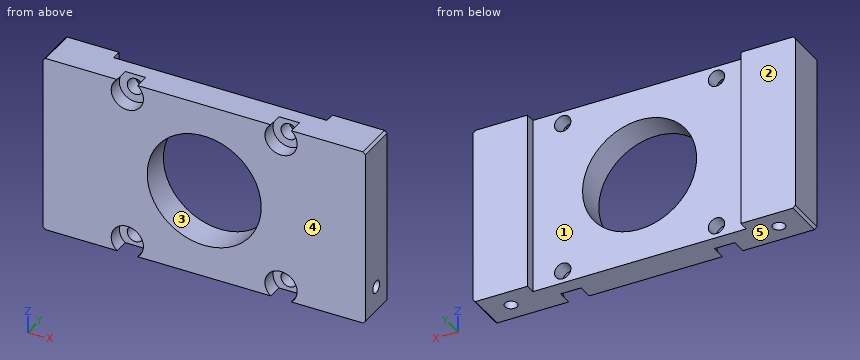
from build123d import *

# Parameters (mm, degrees)
F0_W           = 65
F0_H           = 36
F0_R           = 11.5
F1_DEPTH       = 8
F3_D           = 3.3
F3_CBORE_D     = 6.5
F3_CBORE_DEPTH = 3
F4_SIZE        = 0.5
F6_D           = 2.5
F6_DEPTH       = 13.5
F6_TIP         = 0.7510757738
F7_W           = 43
F7_H           = 36
F7_R           = 1.65
F7_R_2         = 11.5
F8_DEPTH       = 2
F10_D          = 2.5
F10_DEPTH      = 13.5
F10_TIP        = 0.7510757738


with BuildPart() as f1:
    # F0 (on Front) → F1 (new body)
    with BuildSketch(Plane.XZ):
        Rectangle(F0_W, F0_H)
        Circle(F0_R, mode=Mode.SUBTRACT)
    extrude(amount=F1_DEPTH)

    # F3 (through all)
    with Locations(Plane.XZ.offset(8)):
        with Locations((15.5, 15.5), (15.5, -15.5), (-15.5, -15.5), (-15.5, 15.5)):
            CounterBoreHole(F3_D / 2, F3_CBORE_D / 2, F3_CBORE_DEPTH)

    # F4
    f4_edges = [f1.edges().sort_by_distance(p)[0] for p in [
        (-32.5, -4, 18),
        (32.5, -4, 18),
        (32.5, -4, -18),
        (-32.5, -4, -18),
    ]]
    chamfer(f4_edges, length=F4_SIZE)

    # F6
    with Locations(Plane(origin=(0, 0, -18), x_dir=(1, 0, 0), z_dir=(0, 0, -1))):
        with Locations((27, 4), (-27, 4)):
            Hole(F6_D / 2, depth=F6_DEPTH)
            with Locations((0, 0, -(F6_DEPTH + F6_TIP / 2))):  # 118° drill point
                Cone(0, F6_D / 2, F6_TIP, mode=Mode.SUBTRACT)

    # F7 (on face) → F8 (cut)
    with BuildSketch(Plane(origin=(0, 0, 0), x_dir=(-1, 0, 0), z_dir=(0, 1, 0))):
        Rectangle(F7_W, F7_H)
        with Locations((-15.5, -15.5)):
            Circle(F7_R, mode=Mode.SUBTRACT)
        with Locations((15.5, -15.5)):
            Circle(F7_R, mode=Mode.SUBTRACT)
        with Locations((-15.5, 15.5)):
            Circle(F7_R, mode=Mode.SUBTRACT)
        Circle(F7_R_2, mode=Mode.SUBTRACT)
        with Locations((15.5, 15.5)):
            Circle(F7_R, mode=Mode.SUBTRACT)
    extrude(amount=-F8_DEPTH, mode=Mode.SUBTRACT)

    # F10
    with Locations(Plane.YZ.offset(32.5)):
        with Locations((-4, -12.5)):
            Hole(F10_D / 2, depth=F10_DEPTH)
            with Locations((0, 0, -(F10_DEPTH + F10_TIP / 2))):  # 118° drill point
                Cone(0, F10_D / 2, F10_TIP, mode=Mode.SUBTRACT)


solid = f1.part
Could you check a few things on this model? Use its own coordinates, in mm. Face numbers are marked on the shaded views. A direction names the side the tool comes from. Round coordinates to 2 decimals unless told otherwise and drop trailing zeros. Order: outer loops, then holes, each group sorted by start corner. A loop starts at its lowest first (then second) coordinate and runs counter-clockwise, first axis right, second up.
Q1. Imagine slicing it at A-A, the plane z = -15.5. List the corners of the cut face in (x, y) for me, then the cut area to 3 significant figures.
Geometry says:
outline: (-32.5, -8) - (-18.75, -8) - (-18.75, -5) - (-17.15, -5) - (-17.15, -2) - (-21.5, -2) - (-21.5, 0) - (-32.5, 0) - close; (-13.85, -5) - (-12.25, -5) - (-12.25, -8) - (12.25, -8) - (12.25, -5) - (13.85, -5) - (13.85, -2) - (-13.85, -2) - close; (17.15, -5) - (18.75, -5) - (18.75, -8) - (32.5, -8) - (32.5, 0) - (21.5, 0) - (21.5, -2) - (17.15, -2) - close; hole circle Ø2.5 at (-27, -4); hole circle Ø2.5 at (27, -4)
area: 365 mm2
Q2. Imagine slicing it at C-C, the plane x = 15.5. List the corners of the cut face in (y, z) for me.
Geometry says:
outline: (-8, -12.25) - (-5, -12.25) - (-5, -13.85) - (-2, -13.85) - (-2, 13.85) - (-5, 13.85) - (-5, 12.25) - (-8, 12.25) - close; (-5, -18) - (-2, -18) - (-2, -17.15) - (-5, -17.15) - close; (-5, 17.15) - (-2, 17.15) - (-2, 18) - (-5, 18) - close
Q3. Imagine slicing it at B-B, the plane z = 0. List the corners of the cut face in (x, y) for me, then the cut area to 3 significant figures.
Geometry says:
outline: (-32.5, -8) - (-11.5, -8) - (-11.5, -2) - (-21.5, -2) - (-21.5, 0) - (-32.5, 0) - close; (11.5, -8) - (32.5, -8) - (32.5, 0) - (21.5, 0) - (21.5, -2) - (11.5, -2) - close
area: 296 mm2
Q4. Please list where these lines run through material, in increasing order: probe 1 along X at (y, z) = (-6.05, -15.5); probe 2 along Z at (x, y) = (15.5, -4.15); probe 3 along Z at (x, y) = (0, -4.75).
Geometry says:
probe 1: x = -32.5 to -18.75, -12.25 to 12.25, 18.75 to 32.5
probe 2: z = -18 to -17.15, -13.85 to 13.85, 17.15 to 18
probe 3: z = -18 to -11.5, 11.5 to 18
Q5. Thinking about a two-plate mould opening in Z: for the marked faces 3, 4 and 5, which applies, released by +Z, released by -Z, zero draft, split by the parting line, or undercut?
Geometry says:
face 3: undercut
face 4: zero draft
face 5: released by -Z
Q6. I'm going to push flat-ended pins straight in: P1, Ø4.5, axis at x = -15.5, z = 15.5, coming from the -Y side; P2, Ø18, axis at x = 2, z = 5, coming from the +Y side. Where does each tip first touch, or does it pass through?
Geometry says:
P1: stops at y = -5
P2: stops at y = -2
Q7. Which directions (+Z, -Z, +X, -X, +Y, -Y) give clear straight access to the entire face, cutting with the end or side of a thin tool? Please do the marked faces 1 and 2.
Geometry says:
face 1: +Z, -Z, +Y
face 2: +Z, -Z, +X, -X, +Y
Q8. Imagine slicing it at D-D, the plane z = 15.5. List the corners of the cut face in (x, y) for me, then the cut area to 3 significant figures.
Geometry says:
outline: (-32.5, -8) - (-18.75, -8) - (-18.75, -5) - (-17.15, -5) - (-17.15, -2) - (-21.5, -2) - (-21.5, 0) - (-32.5, 0) - close; (-13.85, -5) - (-12.25, -5) - (-12.25, -8) - (12.25, -8) - (12.25, -5) - (13.85, -5) - (13.85, -2) - (-13.85, -2) - close; (17.15, -5) - (18.75, -5) - (18.75, -8) - (32.5, -8) - (32.5, 0) - (21.5, 0) - (21.5, -2) - (17.15, -2) - close
area: 375 mm2
